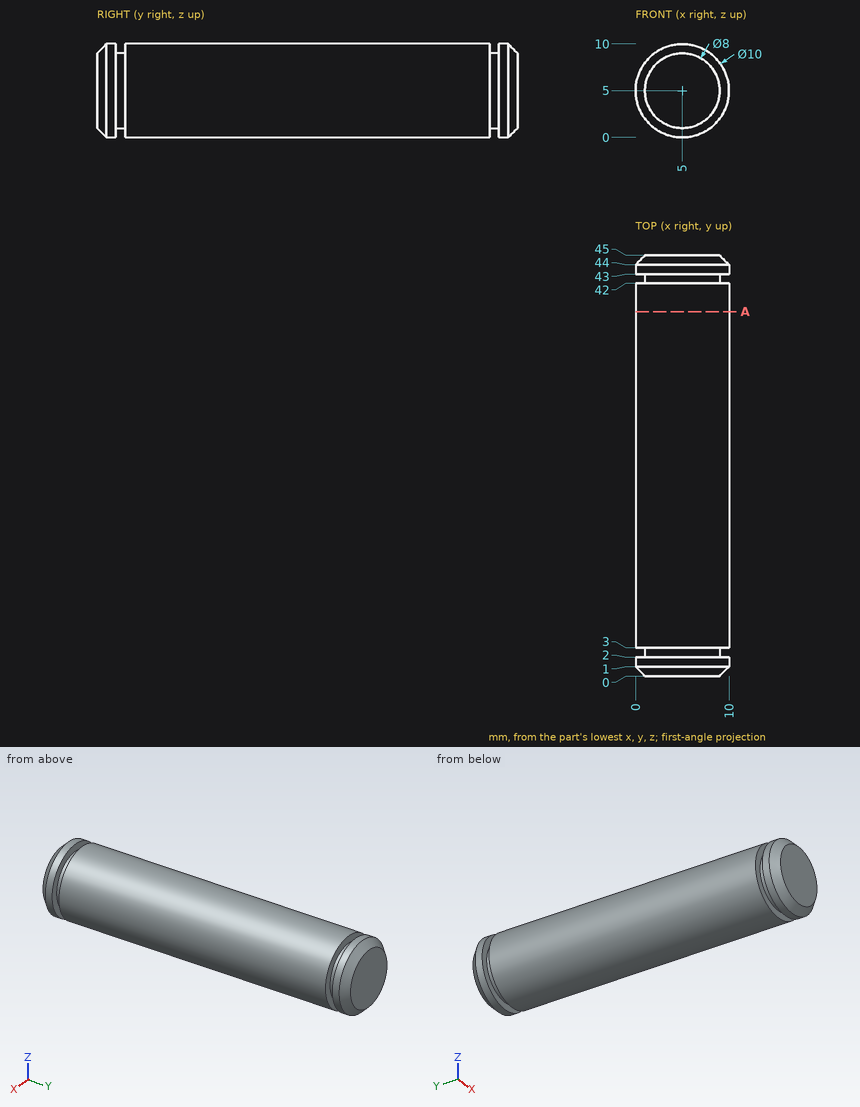
For this review, use the dimensioned drawing (mm, ordinates from the lowest corner) and the shaded views. Give positions to 0.01 mm unless a question says otherwise; leave off trailing zeros. Write each loop counter-clockwise with the first axis right and the second up, starting at its lowest first coordinate (ties: lowest second). Pieces come first, ordered by that corner, then holes.
(1) For P1, Ø4, axis at x = 1, y = 10, coming from the -Z side; P2, Ø1.5, axis at y = 18, z = 7.5, coming from the +X side; P3, Ø6, axis at x = 9, y = 27, coming from the -Z side, all flat-tipped, find the tip position at first contact; note any pin that passes through.
(2) Consider section A-A, the plane y = 39. Give the boundary of the cut face in (x, z), and give its area (3 significant figures).
(3) To check wall thickness, follow L1, parallel to Y at x = 1.5, z = 7.75; L2, parallel to Y at x = 9, z = 2.5; L3, parallel to Z at x = 8, y = 22.5. State the ranges of each line that lie inside material, in increasing order.
Returned:
1. P1: stops at z = 0.42
1. P2: stops at x = 9.68
1. P3: stops at z = 0.1
2. outline: circle Ø10 at (5, 5)
2. area: 78.5 mm2
3. L1: y = 0.45 to 2, 3 to 42, 43 to 44.55
3. L2: y = 0.72 to 2, 3 to 42, 43 to 44.28
3. L3: z = 1 to 9
